Can you work these out from the drawing? Everything is in mm from the part's minimum corner. A direction names the side the tool comes from. Coordinates: 2 decimals unless noted, no trailing zeros. Order: outer loops, then holes, each group sorted by start corner. A loop starts at its lowest first (then second) coordinate and runs counter-clockwise, first axis right, second up. Notation, with made-up numbers: (11, -35.5) - (62, -35.5) arc R31 ccw to (62, 3.5) - close; hole circle Ø7 at (26, 24.5). An arc over 180 degrees is marked (long way). Use a Markdown table: item, result. Add a question column.
(1) For pin 1 Ø3 at (x, y) = (1.5, 3) entering from -Z; pin 2 Ø1.5 at (x, z) = (2.5, 6) entering from -Y; pin 3 Ø2 at (x, z) = (6, 4) entering from +Y, each with a flat end and sliding along its axis, tell me the tip position at first contact or that it passes through.
(2) I want a section at A-A (z = 8.25). List the corners of the cut face in (x, y) for me.
(3) If I drill on L1, parallel to Z at x = 3.5, y = 6.75; L2, parallel to Y at x = 4.5, z = 3.25; L3, parallel to Y at x = 6, z = 4, over which ranges is the centre line in solid material (lowest first)? Write a range as [from, to].
(4) On a 3-axis mill with a long thin cutter (end or side, diameter ignored), from which of +Z, -Z, +X, -X, +Y, -Y can I reach the whole of each face in a straight line? I mean the marked faces 1 and 2. Say none if no direction works.
(5) I want a section at B-B (z = 4). List the corners of the cut face in (x, y) for me.
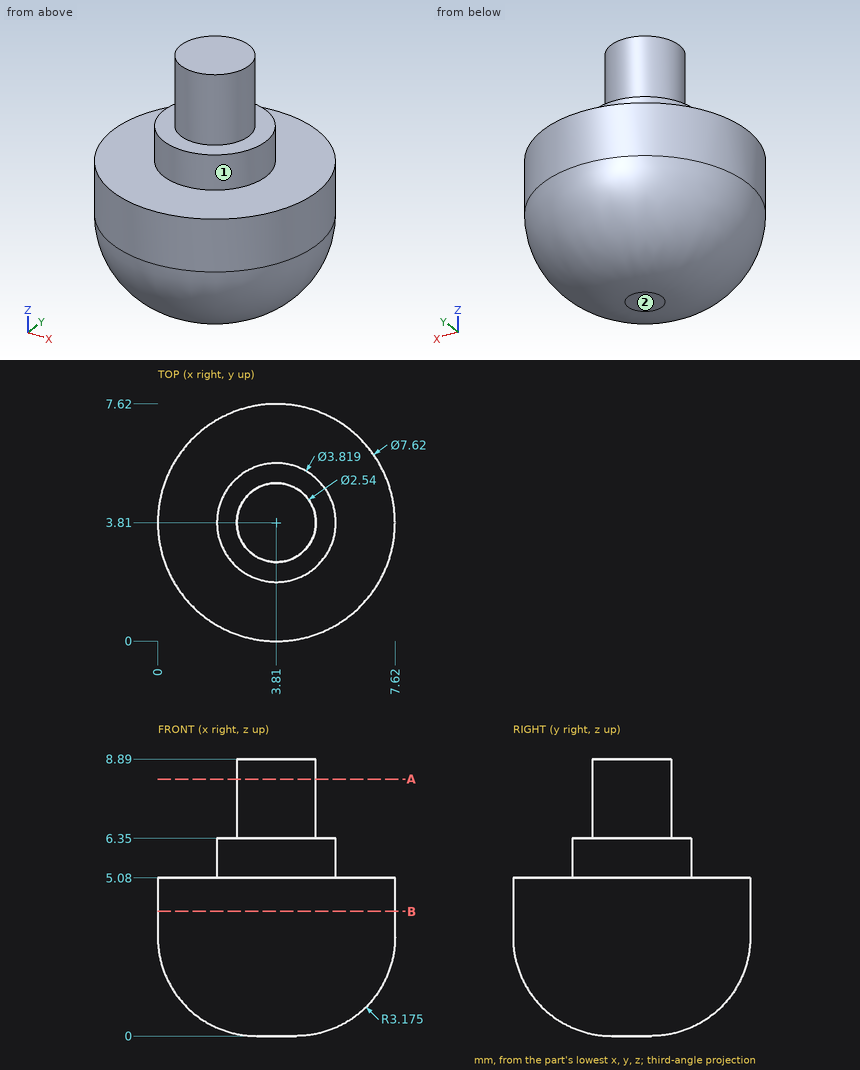
Answers follow:
| question | item | result |
|---|---|---|
| 1 | pin 1 | stops at z = 0.02 |
| 1 | pin 2 | stops at y = 1.98 |
| 1 | pin 3 | stops at y = 7.43 |
| 2 | outline | circle Ø2.54 at (3.81, 3.81) |
| 3 | L1 | z = [1.01, 5.08] |
| 3 | L2 | y = [0.06, 7.56] |
| 3 | L3 | y = [0.69, 6.93] |
| 4 | face 1 | +Z |
| 4 | face 2 | -Z, +X, -X, +Y, -Y |
| 5 | outline | circle Ø7.62 at (3.81, 3.81) |
